```python
from build123d import *

# Parameters (mm, degrees)
SKETCH1_W            = 220
SKETCH1_H            = 150
BOSS_EXTRUDE1_DEPTH  = 3.175
M3_CLEARANCE_HOLE1_D = 3.6
SKETCH4_W            = 10
SKETCH4_H            = 10
BOSS_EXTRUDE2_DEPTH  = 3.175
FILLET2_R            = 1.5
SKETCH7_W            = 30
SKETCH7_H            = 15
CUT_EXTRUDE2_DEPTH   = 4.175
M3_CLEARANCE_HOLE3_D = 3.6
FILLET3_R            = 2


with BuildPart() as part:
    # Sketch1 → Boss-Extrude1 (new body)
    with BuildSketch(Plane.XY):
        Rectangle(SKETCH1_W, SKETCH1_H)
    extrude(amount=BOSS_EXTRUDE1_DEPTH)

    # M3 Clearance Hole1 (through all)
    with Locations(Plane.XY.offset(3.175)):
        with Locations((0, 0), (-80, 70), (80, 70), (0, 70), (-105, 55), (-105, 0), (-105, -55), (-80, -70), (0, -70), (80, -70), (105, -55), (105, 0), (105, 55)):
            Hole(M3_CLEARANCE_HOLE1_D / 2)

    # Sketch4 → Boss-Extrude2 (add, through all)
    with BuildSketch(Plane.XY.offset(3.175)):
        Rectangle(SKETCH4_W, SKETCH4_H)
    extrude(amount=-BOSS_EXTRUDE2_DEPTH)

    # Fillet2
    fillet2_edges = [part.edges().sort_by_distance(p)[0] for p in [
        (-110, -75, 1.5875),
        (-110, 75, 1.5875),
        (110, 75, 1.5875),
        (110, -75, 1.5875),
    ]]
    fillet(fillet2_edges, radius=FILLET2_R)

    # Sketch7 → Cut-Extrude2 (cut, through all)
    with BuildSketch(Plane.XY.offset(3.175)):
        with Locations((-80, 53.5)):
            Rectangle(SKETCH7_W, SKETCH7_H)
    extrude(amount=-CUT_EXTRUDE2_DEPTH, mode=Mode.SUBTRACT)

    # M3 Clearance Hole3 (through all)
    with Locations(Plane.XY.offset(3.175)):
        with Locations((-22.5, 53.5), (22.5, 53.5)):
            Hole(M3_CLEARANCE_HOLE3_D / 2)

    # Fillet3
    fillet3_edges = [part.edges().sort_by_distance(p)[0] for p in [
        (-65, 61, 1.5875),
        (-65, 46, 1.5875),
        (-95, 46, 1.5875),
        (-95, 61, 1.5875),
    ]]
    fillet(fillet3_edges, radius=FILLET3_R)


solid = part.part
```
Part model, mm, in its own coordinate system. Round coordinates to 2 decimals unless told otherwise and drop trailing zeros.
1. Drill centre lines: line 1 along X through (y, z) = (70, 1.55); line 2 along Y through (x, z) = (105, 0.9); line 3 along Y through (x, z) = (0, 0.95). Where is each one in solid material? Low to high.
Solutions:
line 1: x = -110 to -81.8, -78.2 to -1.8, 1.8 to 78.2, 81.8 to 110
line 2: y = -75 to -56.8, -53.2 to -1.8, 1.8 to 53.2, 56.8 to 75
line 3: y = -75 to -71.8, -68.2 to 68.2, 71.8 to 75
2. Flat gauge pins, fed straight in: pin 1 (6 mm diameter, centred on x = 80, y = 70, fed in from -Z); pin 2 (3 mm diameter, centred on x = 105, y = 55, fed in from +Z). Where does each tip first touch, or does it go through?
Solutions:
pin 1: stops at z = 0
pin 2: passes through
3. Slice it at A-A (z = 2.65). Count the separate pieces of the cut face and the enclosed holes in it, and give its area (3 significant figures).
Solutions:
separate pieces: 1
enclosed holes: 15
area: 32,400 mm2
